from build123d import *

# Parameters (mm, degrees)
SKETCH_1_W          = 10
SKETCH_1_H          = 10
EXTRUDE_1_DEPTH     = 300
SKETCH_2_R          = 2.5
CUT_EXTRUDE_1_DEPTH = 301.333148354


with BuildPart() as part:
    # ｽｹｯﾁ1 → ﾎﾞｽ - 押し出し1 (new body)
    with BuildSketch(Plane.XY):
        with Locations((5, -5)):
            Rectangle(SKETCH_1_W, SKETCH_1_H)
    extrude(amount=EXTRUDE_1_DEPTH)

    # ｽｹｯﾁ2 → ｶｯﾄ - 押し出し1 (cut, through all)
    with BuildSketch(Plane(origin=(10, 0, 0), x_dir=(0, 0, -1), z_dir=(1, 0, 0))):
        with Locations(Location((-6, -5, 0), (0, 0, 90))):
            Circle(SKETCH_2_R)
        with Locations(Location((-294, -5, 0), (0, 0, 270))):
            Circle(SKETCH_2_R)
        Polygon((-2.828427125, 0), (0, -2.828427125), (0, 0), align=None)
        Polygon((0, -7.171572875), (-2.828427125, -10), (0, -10), align=None)
        Polygon((-300, 0), (-297.171572875, 0), (-300, -2.828427125), align=None)
        Polygon((-300, -10), (-300, -7.171572875), (-297.171572875, -10), align=None)
    extrude(amount=-CUT_EXTRUDE_1_DEPTH, mode=Mode.SUBTRACT)


solid = part.part
Source: CAD feature listing. Evaluate the final solid. Frame: model axes, mm. Round coordinates to 2 decimals unless told otherwise and drop trailing zeros. Order: outer loops, then holes, each group sorted by start corner. A loop starts at its lowest first (then second) coordinate and runs counter-clockwise, first axis right, second up. Notation, with made-up numbers: (50, -19.75) - (77, -19.75) arc R13 ccw to (77, -14.75) - close; hole circle Ø1 at (60.5, 3.25). An arc over 180 degrees is marked (long way). Use a Markdown table: item, result. Add a question column.
1. First-contact query: pin 1 (5 mm diameter, centred on x = 6.5, y = -5.5, fed in from -Z); pin 2 (4.5 mm diameter, centred on y = -5, z = 294, fed in from +X). Flat tips, straight axial feed; report the tip coordinate or a pass-through.
2. Mould query, pull axis Z, two halves, no side actions, for faces 1 (the cylindrical face through (5.07, -4.67, 291.52)), 2 (the flat face through (0, -5, 148)). Classes: +Z half, -Z half, draft (parallel to the pull), parting line (faces both ways), or undercut.
3. Section query A-A (y = -5). Return the cut outline in (x, z).
4. Section query B-B (x = 2). Return the cut outline in (y, z), then the cut area to 3 significant figures.
5. Section query C-C (z = 294). Return the cut outline in (x, y).
6. Line query: probe 1 along Z at (x, y) = (3, -5); probe 2 along Y at (x, z) = (2, 294); probe 3 along Z at (x, y) = (5.5, -6.25). Output: solid intervals per line, ascending.
Derived:
| question | item | result |
|---|---|---|
| 1 | pin 1 | z = 0 |
| 1 | pin 2 | through |
| 2 | face 1 | undercut |
| 2 | face 2 | draft |
| 3 | outline | (0, 0) - (10, 0) - (10, 3.5) - (0, 3.5) - close; (0, 8.5) - (10, 8.5) - (10, 291.5) - (0, 291.5) - close; (0, 296.5) - (10, 296.5) - (10, 300) - (0, 300) - close |
| 4 | outline | (-10, 2.83) - (-7.17, 0) - (-2.83, 0) - (0, 2.83) - (0, 297.17) - (-2.83, 300) - (-7.17, 300) - (-10, 297.17) - close; hole circle Ø5 at (-5, 6); hole circle Ø5 at (-5, 294) |
| 4 | area | 2,940 mm2 |
| 5 | outline | (0, -10) - (10, -10) - (10, -7.5) - (0, -7.5) - close; (0, -2.5) - (10, -2.5) - (10, 0) - (0, 0) - close |
| 6 | probe 1 | 0 to 3.5, 8.5 to 291.5, 296.5 to 300 |
| 6 | probe 2 | -10 to -7.5, -2.5 to 0 |
| 6 | probe 3 | 0 to 3.83, 8.17 to 291.83, 296.17 to 300 |
